from build123d import *

# Parameters (mm, degrees)
SKETCH_1_R          = 2.65
SKETCH_1_R_2        = 16.5
SKETCH_1_R_3        = 1.25
EXTRUDE_1_DEPTH     = 8
SKETCH_1_3_R        = 16.5
SKETCH_1_3_R_2      = 11
EXTRUDE_2_DEPTH     = 7.5
SKETCH_1_4_R        = 11
SKETCH_1_4_R_2      = 3.65
EXTRUDE_3_DEPTH     = 10
EXTRUDE_4_DEPTH     = 2.6
SKETCH_2_R          = 8
CUT_EXTRUDE_1_DEPTH = 8.6
FILLET_1_R          = 2
FILLET_2_R          = 0.5
CHAMFER_1_SIZE      = 0.3


with BuildPart() as part:
    # Sketch 1 → Extrude 1 (new body)
    with BuildSketch(Plane(origin=(0, 0, 0), x_dir=(1, 0, 0), z_dir=(0, 1, 0))):
        with BuildLine():
            ThreePointArc((-14.600256847, 21.15), (-18.172644276, 18.172644276), (-21.15, 14.600256847))
            Line((-21.15, 14.600256847), (-21.15, -14.600256847))
            ThreePointArc((-21.15, -14.600256847), (-18.172644276, -18.172644276), (-14.600256847, -21.15))
            Line((-14.600256847, -21.15), (14.600256847, -21.15))
            ThreePointArc((14.600256847, -21.15), (18.172644276, -18.172644276), (21.15, -14.600256847))
            Line((21.15, -14.600256847), (21.15, 14.600256847))
            ThreePointArc((21.15, 14.600256847), (18.172644276, 18.172644276), (14.600256847, 21.15))
            Line((14.600256847, 21.15), (-14.600256847, 21.15))
        make_face()
        with Locations((-15.5, -15.5)):
            Circle(SKETCH_1_R, mode=Mode.SUBTRACT)
        with Locations((15.5, -15.5)):
            Circle(SKETCH_1_R, mode=Mode.SUBTRACT)
        Circle(SKETCH_1_R_2, mode=Mode.SUBTRACT)
        with Locations((-15.5, 15.5)):
            Circle(SKETCH_1_R, mode=Mode.SUBTRACT)
        with Locations((15.5, 15.5)):
            Circle(SKETCH_1_R, mode=Mode.SUBTRACT)
        with Locations((15.5, -15.5)):
            Circle(SKETCH_1_R)
        with Locations((15.5, -15.5)):
            Circle(SKETCH_1_R_3, mode=Mode.SUBTRACT)
        with Locations((-15.5, -15.5)):
            Circle(SKETCH_1_R)
        with Locations((-15.5, -15.5)):
            Circle(SKETCH_1_R_3, mode=Mode.SUBTRACT)
        with Locations((-15.5, 15.5)):
            Circle(SKETCH_1_R)
        with Locations((-15.5, 15.5)):
            Circle(SKETCH_1_R_3, mode=Mode.SUBTRACT)
        with Locations((15.5, 15.5)):
            Circle(SKETCH_1_R)
        with Locations((15.5, 15.5)):
            Circle(SKETCH_1_R_3, mode=Mode.SUBTRACT)
        with BuildLine():
            ThreePointArc((-14.600256847, -21.15), (-18.172644276, -18.172644276), (-21.15, -14.600256847))
            Line((-21.15, -14.600256847), (-21.15, -17.35))
            Line((-21.15, -17.35), (-17.35, -21.15))
            Line((-17.35, -21.15), (-14.600256847, -21.15))
        make_face()
        with BuildLine():
            Line((-17.35, 21.15), (-21.15, 17.35))
            Line((-21.15, 17.35), (-21.15, 14.600256847))
            ThreePointArc((-21.15, 14.600256847), (-18.172644276, 18.172644276), (-14.600256847, 21.15))
            Line((-14.600256847, 21.15), (-17.35, 21.15))
        make_face()
        with BuildLine():
            Line((17.35, 21.15), (14.600256847, 21.15))
            ThreePointArc((14.600256847, 21.15), (18.172644276, 18.172644276), (21.15, 14.600256847))
            Line((21.15, 14.600256847), (21.15, 17.35))
            Line((21.15, 17.35), (17.35, 21.15))
        make_face()
        with BuildLine():
            ThreePointArc((21.15, -14.600256847), (18.172644276, -18.172644276), (14.600256847, -21.15))
            Line((14.600256847, -21.15), (17.35, -21.15))
            Line((17.35, -21.15), (21.15, -17.35))
            Line((21.15, -17.35), (21.15, -14.600256847))
        make_face()
    extrude(amount=EXTRUDE_1_DEPTH)

    # Sketch 1_3 → Extrude 2 (add)
    with BuildSketch(Plane(origin=(0, 0, 0), x_dir=(1, 0, 0), z_dir=(0, 1, 0))):
        Circle(SKETCH_1_3_R)
        Circle(SKETCH_1_3_R_2, mode=Mode.SUBTRACT)
    extrude(amount=EXTRUDE_2_DEPTH)

    # Sketch 1_4 → Extrude 3 (add)
    with BuildSketch(Plane(origin=(0, 0, 0), x_dir=(1, 0, 0), z_dir=(0, 1, 0))):
        Circle(SKETCH_1_4_R)
        Circle(SKETCH_1_4_R_2, mode=Mode.SUBTRACT)
    extrude(amount=EXTRUDE_3_DEPTH)

    # Sketch 1_5 → Extrude 4 (add)
    with BuildSketch(Plane(origin=(0, 0, 0), x_dir=(1, 0, 0), z_dir=(0, 1, 0))):
        with BuildLine():
            ThreePointArc((-14.600256847, -21.15), (-18.172644276, -18.172644276), (-21.15, -14.600256847))
            Line((-21.15, -14.600256847), (-21.15, -17.35))
            Line((-21.15, -17.35), (-17.35, -21.15))
            Line((-17.35, -21.15), (-14.600256847, -21.15))
        make_face()
        with BuildLine():
            ThreePointArc((21.15, -14.600256847), (18.172644276, -18.172644276), (14.600256847, -21.15))
            Line((14.600256847, -21.15), (17.35, -21.15))
            Line((17.35, -21.15), (21.15, -17.35))
            Line((21.15, -17.35), (21.15, -14.600256847))
        make_face()
        with BuildLine():
            Line((-17.35, 21.15), (-21.15, 17.35))
            Line((-21.15, 17.35), (-21.15, 14.600256847))
            ThreePointArc((-21.15, 14.600256847), (-18.172644276, 18.172644276), (-14.600256847, 21.15))
            Line((-14.600256847, 21.15), (-17.35, 21.15))
        make_face()
        with BuildLine():
            Line((17.35, 21.15), (14.600256847, 21.15))
            ThreePointArc((14.600256847, 21.15), (18.172644276, 18.172644276), (21.15, 14.600256847))
            Line((21.15, 14.600256847), (21.15, 17.35))
            Line((21.15, 17.35), (17.35, 21.15))
        make_face()
    extrude(amount=-EXTRUDE_4_DEPTH)

    # Sketch 2 → Cut-Extrude 1 (cut)
    with BuildSketch(Plane.XZ):
        Circle(SKETCH_2_R)
    extrude(amount=-CUT_EXTRUDE_1_DEPTH, mode=Mode.SUBTRACT)

    # Fillet 1
    fillet_1_edges = [part.edges().sort_by_distance(p)[0] for p in [
        (-17.35, 2.7, 21.15),
        (-21.15, 2.7, 17.35),
        (-21.15, 2.7, -17.35),
        (-17.35, 2.7, -21.15),
        (17.35, 2.7, -21.15),
        (21.15, 2.7, -17.35),
        (21.15, 2.7, 17.35),
        (17.35, 2.7, 21.15),
    ]]
    fillet(fillet_1_edges, radius=FILLET_1_R)

    # Fillet 2
    fillet_2_edges = [part.edges().sort_by_distance(p)[0] for p in [
        (21.15, 8, 0),
        (19.25, 8, 19.25),
        (0, 8, 21.15),
        (19.25, 8, -19.25),
        (0, 8, -21.15),
        (-19.25, 8, -19.25),
        (-21.15, 8, 0),
        (-19.25, 8, 19.25),
        (20.997759065, 8, -17.28693974),
        (17.28693974, 8, -20.997759065),
        (-17.28693974, 8, -20.997759065),
        (-20.997759065, 8, -17.28693974),
        (-20.997759065, 8, 17.28693974),
        (-17.28693974, 8, 20.997759065),
        (17.28693974, 8, 20.997759065),
        (20.997759065, 8, 17.28693974),
        (-3.65, 10, 0),
        (-11, 10, 0),
    ]]
    fillet(fillet_2_edges, radius=FILLET_2_R)

    # Chamfer 1
    chamfer_1_edges = [part.edges().sort_by_distance(p)[0] for p in [
        (-16.75, 8, -15.5),
        (14.25, 8, -15.5),
        (14.25, 8, 15.5),
        (-16.75, 8, 15.5),
    ]]
    chamfer(chamfer_1_edges, length=CHAMFER_1_SIZE)


solid = part.part
Geometry: final body of the model. Coordinates: model frame, mm. A direction names the side the tool comes from. Round coordinates to 2 decimals unless told otherwise and drop trailing zeros. Loops run counter-clockwise (first coordinate to the right, second up) from the corner with the lowest first, then second, coordinate; pieces in that order, holes last. Notation, with made-up numbers: M 55.25,13 L 107.25,13 A21 cw 107.25,19 Z; hole C 10,82.5 d2. An arc over 180 degrees is marked long. Put each result on its own line as item: value. Start each with the question number.
(1) Set-up query: faces 5 (the face through (-2.38, 8.49, 10.74)), 6 (the face through (18.126, -1.282, -18.219)), 7 (the face through (3.48, 9.04, -1.1)). Return all of +Z, -Z, +X, -X, +Y, -Y with unobstructed straight access to the full face (end or side cutting, diameter ignored); none if empty.
(2) Material intervals for line 1 along X through (y, z) = (4.5, -15.5); line 2 along Z through (x, y) = (0, 3.5), sorted ascending. Write a range as [from, to].
(3) Draft query along X for faces 1 (the face through (-1.73, 4.24, -7.81)), 2 (the face through (-21, 2.38, -17.28)), 3 (the face through (20.994, 2.379, 17.297)), 4 (the face through (15.24, 7.75, 6.32)). Return one class per face: +X half, -X half, draft (parallel to the pull), parting line (faces both ways), or undercut.
(4) Section query A-A (x = 0). Return loops of the section in (y, z).
(5) Contact query for flat-ended pins moving along their axis: pin 1 Ø6 at (x, z) = (-0.5, 12) entering from -Y; pin 2 Ø2 at (x, z) = (10, -15.5) entering from +Y; pin 3 Ø9.5 at (x, z) = (0, 0) entering from +Y. Output: stop coordinate, or through.
(6) Section query D-D (x = 15.5). Return loops of the section in (y, z).
(7) Section query B-B (z = 0). Return loops of the section in (x, y).
(8) Section query C-C (y = 5.5). Return loops of the section in (x, z).
Findings below:
1. face 5: +Y
1. face 6: -Y
1. face 7: +Y, -Y
2. line 1: x = [-21.15, -16.75], [-14.25, 14.25], [16.75, 21.15]
2. line 2: z = [-21.15, -8], [8, 21.15]
3. face 1: undercut
3. face 2: -X half
3. face 3: +X half
3. face 4: undercut
4. outline: M 0,-21.15 L 7.5,-21.15 A0.5 ccw 8,-20.65 L 8,-16.5 L 7.5,-16.5 L 7.5,-11 L 9.5,-11 A0.5 ccw 10,-10.5 L 10,-4.15 A0.5 ccw 9.5,-3.65 L 8.6,-3.65 L 8.6,-8 L 0,-8 Z; M 0,8 L 8.6,8 L 8.6,3.65 L 9.5,3.65 A0.5 ccw 10,4.15 L 10,10.5 A0.5 ccw 9.5,11 L 7.5,11 L 7.5,16.5 L 8,16.5 L 8,20.65 A0.5 ccw 7.5,21.15 L 0,21.15 Z
5. pin 1: stops at y = 0
5. pin 2: stops at y = 8
5. pin 3: stops at y = 10
6. outline: M -2.6,-21.15 L 7.5,-21.15 A0.5 ccw 8,-20.65 L 8,-17.05 L 7.7,-16.75 L 0,-16.75 L 0,-20.5 L -2.6,-20.5 Z; M -2.6,20.5 L 0,20.5 L 0,16.75 L 7.7,16.75 L 8,17.05 L 8,20.65 A0.5 ccw 7.5,21.15 L -2.6,21.15 Z; M 0,-14.25 L 7.7,-14.25 L 8,-13.95 L 8,-5.66 L 7.5,-5.66 L 7.5,5.66 L 8,5.66 L 8,13.95 L 7.7,14.25 L 0,14.25 Z
7. outline: M -21.15,0 L -8,0 L -8,8.6 L -3.65,8.6 L -3.65,9.5 A0.5 ccw -4.15,10 L -10.5,10 A0.5 ccw -11,9.5 L -11,7.5 L -16.5,7.5 L -16.5,8 L -20.65,8 A0.5 ccw -21.15,7.5 Z; M 3.65,8.6 L 8,8.6 L 8,0 L 21.15,0 L 21.15,7.5 A0.5 ccw 20.65,8 L 16.5,8 L 16.5,7.5 L 11,7.5 L 11,9.5 A0.5 ccw 10.5,10 L 4.15,10 A0.5 ccw 3.65,9.5 Z
8. outline: M -21.15,-16.52 A2 ccw -20.56,-17.94 L -17.94,-20.56 A2 ccw -16.52,-21.15 L 16.52,-21.15 A2 ccw 17.94,-20.56 L 20.56,-17.94 A2 ccw 21.15,-16.52 L 21.15,16.52 A2 ccw 20.56,17.94 L 17.94,20.56 A2 ccw 16.52,21.15 L -16.52,21.15 A2 ccw -17.94,20.56 L -20.56,17.94 A2 ccw -21.15,16.52 Z; hole C -15.5,-15.5 d2.5; hole C -15.5,15.5 d2.5; hole C 0,0 d16; hole C 15.5,-15.5 d2.5; hole C 15.5,15.5 d2.5
